```python
from build123d import *

# Parameters (mm, degrees)
SKETCH_W        = 60
SKETCH_H        = 30
PAD_DEPTH       = 20
SKETCH001_W     = 14
SKETCH001_H     = 5
POCKET_DEPTH    = 20.001
SKETCH002_W     = 14
SKETCH002_H     = 5
POCKET001_DEPTH = 20.001
SKETCH003_W     = 38
SKETCH003_H     = 20
POCKET002_DEPTH = 20.001
SKETCH005_W     = 38
SKETCH005_H     = 5
POCKET003_DEPTH = 20.001
SKETCH006_W     = 9
SKETCH006_H     = 3
POCKET004_DEPTH = 20.001
SKETCH007_W     = 1
SKETCH007_H     = 4
POCKET005_DEPTH = 20.001
SKETCH008_W     = 30
SKETCH008_H     = 18
POCKET006_DEPTH = 5
FILLET_R        = 1
FILLET001_R     = 1
FILLET002_R     = 1
FILLET003_R     = 1
FILLET004_R     = 1
FILLET005_R     = 1
FILLET006_R     = 1
FILLET007_R     = 1
SKETCH011_W     = 20
SKETCH011_H     = 18
POCKET007_DEPTH = 10
SKETCH012_W     = 20
SKETCH012_H     = 18
POCKET008_DEPTH = 10
FILLET008_R     = 1
FILLET009_R     = 1
SKETCH014_W     = 6
SKETCH014_H     = 10
POCKET009_DEPTH = 60.001
SKETCH015_R     = 1.5
POCKET010_DEPTH = 5
SKETCH016_R     = 1.5
POCKET011_DEPTH = 60.001


with BuildPart() as part:
    # Sketch → Pad (new body)
    with BuildSketch(Plane.XZ):
        with Locations((30, 15)):
            Rectangle(SKETCH_W, SKETCH_H)
    extrude(amount=PAD_DEPTH)

    # Sketch001 (on Face6 of Pad) → Pocket (cut, through all)
    with BuildSketch(Plane.XZ.offset(20)):
        with Locations((8, 3.5)):
            Rectangle(SKETCH001_W, SKETCH001_H)
    extrude(amount=-POCKET_DEPTH, mode=Mode.SUBTRACT)

    # Sketch002 (on Face5 of Pocket) → Pocket001 (cut, through all)
    with BuildSketch(Plane.XZ.offset(20)):
        with Locations((52, 3.5)):
            Rectangle(SKETCH002_W, SKETCH002_H)
    extrude(amount=-POCKET001_DEPTH, mode=Mode.SUBTRACT)

    # Sketch003 (on Face5 of Pocket001) → Pocket002 (cut, through all)
    with BuildSketch(Plane.XZ.offset(20)):
        with Locations((30, 16)):
            Rectangle(SKETCH003_W, SKETCH003_H)
    extrude(amount=-POCKET002_DEPTH, mode=Mode.SUBTRACT)

    # Sketch005 (on Face5 of Pocket002) → Pocket003 (cut, through all)
    with BuildSketch(Plane.XZ.offset(20)):
        with Locations((30, 28.5)):
            Rectangle(SKETCH005_W, SKETCH005_H)
    extrude(amount=-POCKET003_DEPTH, mode=Mode.SUBTRACT)

    # Sketch006 (on Face5 of Pocket003) → Pocket004 (cut, through all)
    with BuildSketch(Plane.XZ.offset(20)):
        with Locations((5.5, 27.5)):
            Rectangle(SKETCH006_W, SKETCH006_H)
        with Locations((54.5, 27.5)):
            Rectangle(SKETCH006_W, SKETCH006_H)
    extrude(amount=-POCKET004_DEPTH, mode=Mode.SUBTRACT)

    # Sketch007 (on Face5 of Pocket004) → Pocket005 (cut, through all)
    with BuildSketch(Plane.XZ.offset(20)):
        with Locations((10.5, 28)):
            Rectangle(SKETCH007_W, SKETCH007_H)
        with Locations((49.5, 28)):
            Rectangle(SKETCH007_W, SKETCH007_H)
    extrude(amount=-POCKET005_DEPTH, mode=Mode.SUBTRACT)

    # Sketch008 (on Face18 of Pocket005) → Pocket006 (cut)
    with BuildSketch(Plane(origin=(0, 0, 6), x_dir=(-1, 0, 0), z_dir=(0, 0, 1))):
        with Locations((-30, 10)):
            Rectangle(SKETCH008_W, SKETCH008_H)
    extrude(amount=-POCKET006_DEPTH, mode=Mode.SUBTRACT)

    # Fillet
    fillet_edges = [part.edges().sort_by_distance(p)[0] for p in [
        (60, -10, 0),
    ]]
    fillet(fillet_edges, radius=FILLET_R)

    # Fillet001
    fillet001_edges = [part.edges().sort_by_distance(p)[0] for p in [
        (0, -10, 0),
    ]]
    fillet(fillet001_edges, radius=FILLET001_R)

    # Fillet002
    fillet002_edges = [part.edges().sort_by_distance(p)[0] for p in [
        (0, -10, 30),
    ]]
    fillet(fillet002_edges, radius=FILLET002_R)

    # Fillet003
    fillet003_edges = [part.edges().sort_by_distance(p)[0] for p in [
        (60, -10, 30),
    ]]
    fillet(fillet003_edges, radius=FILLET003_R)

    # Fillet004
    fillet004_edges = [part.edges().sort_by_distance(p)[0] for p in [
        (1, -10, 29),
    ]]
    fillet(fillet004_edges, radius=FILLET004_R)

    # Fillet005
    fillet005_edges = [part.edges().sort_by_distance(p)[0] for p in [
        (1, -10, 1),
    ]]
    fillet(fillet005_edges, radius=FILLET005_R)

    # Fillet006
    fillet006_edges = [part.edges().sort_by_distance(p)[0] for p in [
        (59, -10, 29),
    ]]
    fillet(fillet006_edges, radius=FILLET006_R)

    # Fillet007
    fillet007_edges = [part.edges().sort_by_distance(p)[0] for p in [
        (59, -10, 1),
    ]]
    fillet(fillet007_edges, radius=FILLET007_R)

    # Sketch011 (on Face6 of Fillet007) → Pocket007 (cut)
    with BuildSketch(Plane(origin=(49, 0, 0), x_dir=(0, 0, -1), z_dir=(-1, 0, 0))):
        with Locations((-16, 10)):
            Rectangle(SKETCH011_W, SKETCH011_H)
    extrude(amount=-POCKET007_DEPTH, mode=Mode.SUBTRACT)

    # Sketch012 (on Face21 of Pocket007) → Pocket008 (cut)
    with BuildSketch(Plane(origin=(11, 0, 0), x_dir=(0, 0, 1), z_dir=(1, 0, 0))):
        with Locations((16, 10)):
            Rectangle(SKETCH012_W, SKETCH012_H)
    extrude(amount=-POCKET008_DEPTH, mode=Mode.SUBTRACT)

    # Fillet008
    fillet008_edges = [part.edges().sort_by_distance(p)[0] for p in [
        (30, -19, 1),
    ]]
    fillet(fillet008_edges, radius=FILLET008_R)

    # Fillet009
    fillet009_edges = [part.edges().sort_by_distance(p)[0] for p in [
        (30, -1, 1),
    ]]
    fillet(fillet009_edges, radius=FILLET009_R)

    # Sketch014 (on Face33 of Fillet009) → Pocket009 (cut, through all)
    with BuildSketch(Plane(origin=(60, 0, 0), x_dir=(0, 0, 1), z_dir=(1, 0, 0))):
        with Locations((4, 10)):
            Rectangle(SKETCH014_W, SKETCH014_H)
    extrude(amount=-POCKET009_DEPTH, mode=Mode.SUBTRACT)

    # Sketch015 (on Face32 of Pocket009) → Pocket010 (cut)
    with BuildSketch(Plane(origin=(0, 0, 0), x_dir=(1, 0, 0), z_dir=(0, 0, -1))):
        with Locations((55, 5)):
            Circle(SKETCH015_R)
        with Locations((55, 15)):
            Circle(SKETCH015_R)
        with Locations((5, 5)):
            Circle(SKETCH015_R)
        with Locations((5, 15)):
            Circle(SKETCH015_R)
    extrude(amount=-POCKET010_DEPTH, mode=Mode.SUBTRACT)

    # Sketch016 (on Face30 of Pocket010) → Pocket011 (cut, through all)
    with BuildSketch(Plane(origin=(0, 0, 0), x_dir=(0, 0, -1), z_dir=(-1, 0, 0))):
        with Locations((-15.994056, 9.992209)):
            Circle(SKETCH016_R)
    extrude(amount=-POCKET011_DEPTH, mode=Mode.SUBTRACT)


solid = part.part
```
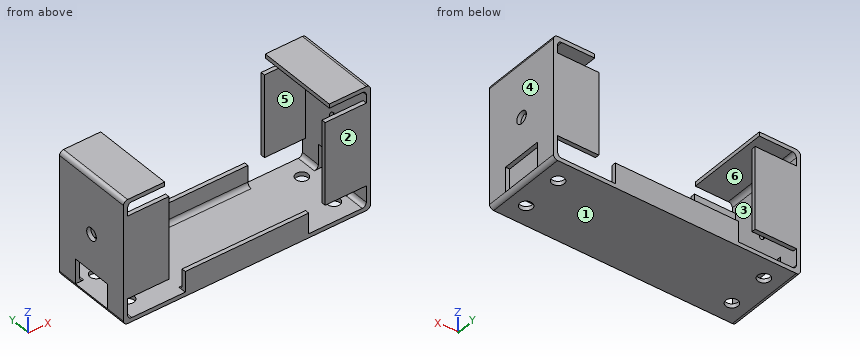
Geometry: final body of the model. Coordinates: model frame, mm. Face numbers are marked on the shaded views. A direction names the side the tool comes from. Round coordinates to 2 decimals unless told otherwise and drop trailing zeros. Order: outer loops, then holes, each group sorted by start corner. A loop starts at its lowest first (then second) coordinate and runs counter-clockwise, first axis right, second up. Notation, with made-up numbers: (64, -36.75) -> (104, -36.75) arc R24 ccw to (104, -5.75) -> close; hole circle Ø9 at (61, -28.5). An arc over 180 degrees is marked (long way). Use one line per item in the form item = value.
(1) Section D-D on x = 35.5. Return loops of the section in (y, z), and give its area (3 significant figures).
Results list:
outline = (-20, 0) -> (0, 0) -> (0, 6) -> (-1, 6) -> (-1, 2) arc R1 cw to (-2, 1) -> (-18, 1) arc R1 cw to (-19, 2) -> (-19, 6) -> (-20, 6) -> close
area = 30.4 mm^2
(2) Section C-C on y = -2.75. Return loops of the section in (x, z).
Results list:
outline = (0, 1) arc R1 ccw to (1, 0) -> (59, 0) arc R1 ccw to (60, 1) -> (60, 29) arc R1 ccw to (59, 30) -> (50, 30) -> (50, 29) -> (58, 29) arc R1 cw to (59, 28) -> (59, 2) arc R1 cw to (58, 1) -> (2, 1) arc R1 cw to (1, 2) -> (1, 28) arc R1 cw to (2, 29) -> (10, 29) -> (10, 30) -> (1, 30) arc R1 ccw to (0, 29) -> close
(3) Section B-B on z = 21. Return loops of the section in (x, y), and give its area (3 significant figures).
Results list:
outline = (0, -20) -> (11, -20) -> (11, -19) -> (1, -19) -> (1, -1) -> (11, -1) -> (11, 0) -> (0, 0) -> close; (49, -20) -> (60, -20) -> (60, 0) -> (49, 0) -> (49, -1) -> (59, -1) -> (59, -19) -> (49, -19) -> close
area = 80.0 mm^2
(4) Section A-A on x = 7.5. Return loops of the section in (y, z), and give its area (3 significant figures).
Results list:
outline = (-20, 0) -> (0, 0) -> (0, 1) -> (-20, 1) -> close; (-20, 6) -> (-19, 6) -> (-19, 26) -> (-20, 26) -> close; (-20, 29) -> (0, 29) -> (0, 30) -> (-20, 30) -> close; (-1, 6) -> (0, 6) -> (0, 26) -> (-1, 26) -> close
area = 80.0 mm^2
(5) Draft query along Y for the marked faces 1, 2 and 3. Return one class per face: pulls with the +Y half, pulls with the -Y half, needs draft (parallel to the pull), parting line crosses it, or undercut.
Results list:
face_1 = needs draft
face_2 = pulls with the -Y half
face_3 = undercut
(6) First-contact query: pin 1 Ø8 at (x, z) = (7, 19.5) entering from +Y; pin 2 Ø2.5 at (x, y) = (55, -15) entering from -Z; pin 3 Ø10 at (x, y) = (26.5, -9) entering from +Z; pin 4 Ø4 at (x, z) = (14.5, 22.5) entering from +Y. Flat tips, straight axial feed; report the tip coordinate or a pass-through.
Results list:
pin_1 = 0
pin_2 = 29
pin_3 = 1
pin_4 = through
(7) Access query for the marked faces 4, 5 and 6. Directions: +Z, -Z, +X, -X, +Y, -Y. A direction counts if a zero-diameter tool reaches every point of the face in a straight line with its end or side. Return the directions, or none.
Results list:
face_4 = +Z, -Z, +X, +Y, -Y
face_5 = none
face_6 = +Y, -Y
(8) Ray query, probe 1 along X at (y, z) = (-5, 0.85); probe 2 along Y at (x, z) = (55, 0.45); probe 3 along Y at (x, z) = (10, 12.5). Return the intervals inside material, ascending. Write a range as [from, to].
Results list:
probe_1 = [0.01, 3.5], [6.5, 53.5], [56.5, 59.99]
probe_2 = [-20, -16.5], [-13.5, -6.5], [-3.5, 0]
probe_3 = [-20, -19], [-1, 0]
